from build123d import *

# Parameters (mm, degrees)
SKETCH1_R           = 4.875
SKETCH1_R_2         = 2.375
BOSS_EXTRUDE1_DEPTH = 17.25
FILLET1_R           = 0.2


with BuildPart() as part:
    # Sketch1 → Boss-Extrude1 (new body)
    with BuildSketch(Plane(origin=(0, 0, 0), x_dir=(1, 0, 0), z_dir=(0, 1, 0))):
        with Locations(Location((0, 0, 0), (0, 0, 270))):
            Circle(SKETCH1_R)
        with Locations(Location((0, 0, 0), (0, 0, 270))):
            Circle(SKETCH1_R_2, mode=Mode.SUBTRACT)
    extrude(amount=BOSS_EXTRUDE1_DEPTH)

    # Sketch3 → Cut-Revolve3 (revolve, cut)
    with BuildSketch(Plane(origin=(0, 15, 0), x_dir=(-1, 0, 0), z_dir=(0, -1, 0))):
        with BuildLine():
            Line((0, 4), (0, -4))
            ThreePointArc((0, -4), (4, 0), (0, 4))
        make_face()
    revolve(axis=Axis((0, 15, -5.147727802), (0, 0, 1)), mode=Mode.SUBTRACT)

    # Fillet1
    fillet1_edges = [part.edges().sort_by_distance(p)[0] for p in [
        (0, 17.25, -3.307189139),
    ]]
    fillet(fillet1_edges, radius=FILLET1_R)


solid = part.part
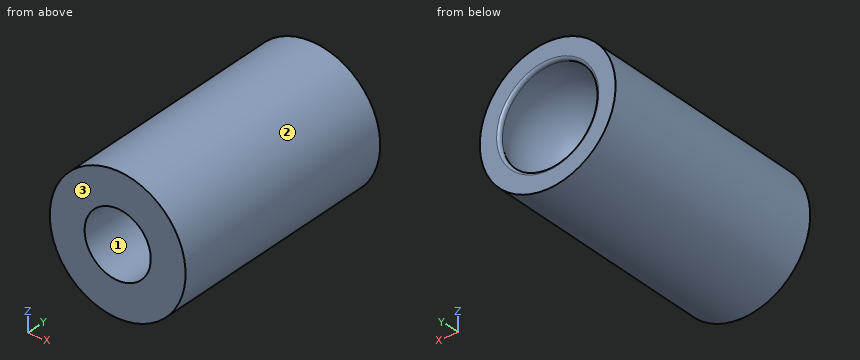
Design review of the part built by this model. Coordinates are the model's own, in mm. Face numbers are marked on the shaded views. Round coordinates to 2 decimals unless told otherwise and drop trailing zeros. Write each loop counter-clockwise with the first axis right and the second up, starting at its lowest first coordinate (ties: lowest second). Pieces come first, ordered by that corner, then holes. Notation, with made-up numbers: (-20.75, -17.75) - (1.25, -17.75) arc R7 ccw to (1.25, -4.75) - close; hole circle Ø3 at (19.25, 14.25). An arc over 180 degrees is marked (long way). Use a Markdown table: item, result. Add a question column.
1. We need section B-B (y = 15.5). State the section outline as (x, z) points (3 decimals), then the cut area to 3 significant figures.
2. Clearance check with flat-ended pins moving along their axes: pin 1 (4 mm diameter, centred on x = 3.5, y = 8.5, fed in from -Z); pin 2 (1.5 mm diameter, centred on x = 1.5, y = 14.5, fed in from +Z); pin 3 (4 mm diameter, centred on y = 4.5, z = 3.5, fed in from +X); pin 4 (4 mm diameter, centred on x = 0, z = 0, fed in from +Y). State where each tip first meets the part, or that it passes through.
3. We need section A-A (y = 4.5). State the section outline as (x, z) points (3 decimals), then the cut area to 3 significant figures.
4. Wall thickness on probe 1 along X at (y, z) = (8.25, 0) (3 decimals); probe 2 along X at (y, z) = (12.5, -2.5); probe 3 along Y at (x, z) = (-3, 2): over which ranges is each line inside the solid? List them lowest first.
5. Mouldability with a two-part tool opening along Z and no side actions: class the marked faces 1, 2 and 3 as +Z half, -Z half, draft (parallel to the pull), parting line (faces both ways), or undercut.
Output:
| question | item | result |
|---|---|---|
| 1 | outline | circle Ø9.75 at (0, 0); hole circle Ø7.937 at (0, 0) |
| 1 | area | 25.2 mm2 |
| 2 | pin 1 | stops at z = -4.64 |
| 2 | pin 2 | stops at z = 4.82 |
| 2 | pin 3 | stops at x = 4.64 |
| 2 | pin 4 | passes through |
| 3 | outline | circle Ø9.75 at (0, 0); hole circle Ø4.75 at (0, 0) |
| 3 | area | 56.9 mm2 |
| 4 | probe 1 | x = -4.875 to -2.375, 2.375 to 4.875 |
| 4 | probe 2 | x = -4.19 to -1.87, 1.87 to 4.19 |
| 4 | probe 3 | y = 0 to 13.27, 16.73 to 17.24 |
| 5 | face 1 | undercut |
| 5 | face 2 | parting line |
| 5 | face 3 | draft |
